Check sheet for the modelled part. Datum: model origin and axes. Units: mm. Give positions to 0.01 mm unless a question says otherwise; leave off trailing zeros. Order: outer loops, then holes, each group sorted by start corner. A loop starts at its lowest first (then second) coordinate and runs counter-clockwise, first axis right, second up. Notation, with made-up numbers: (-37, 37) -> (6, 37) arc R24 cw to (6, 66) -> close; hole circle Ø2 at (63.25, 19.25). An arc over 180 degrees is marked (long way). Write each question's results on one line, items separated by ' | '.
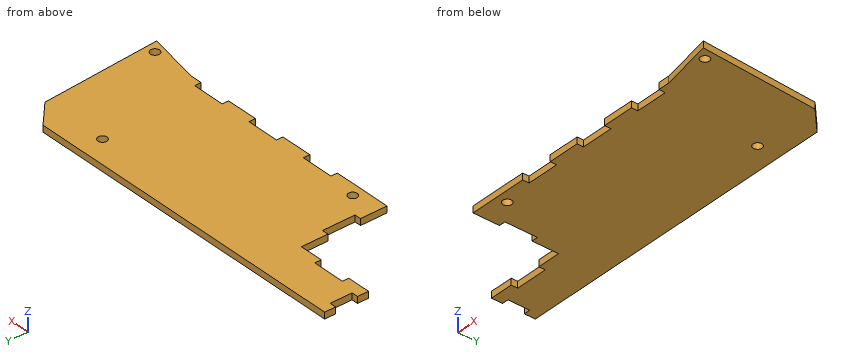
Autodesk Inventor part; units mm, degrees
ref_plane "YZ Plane" through (0, 0, 0) normal (1, 0, 0) x (0, 1, 0)
ref_plane "XZ Plane" through (0, 0, 0) normal (0, 1, 0) x (-1, 0, 0)
ref_plane "XY Plane" through (0, 0, 0) normal (0, 0, 1) x (1, 0, 0)
sketch "Sketch1" plane through (0, 0, 0) normal (0, 0, 1) x (1, 0, 0)
  line L0 (-66.5, -32.75) -> (66.5, -32.75)
  line L1 (66.5, -32.75) -> (66.5, 32.75)
  line L2 (66.5, 32.75) -> (-66.5, 32.75)
  line L3 (-66.5, 32.75) -> (-66.5, -32.75)
  line L4 (-66.5, -32.75) -> (66.5, 32.75) construction
  line L5 (66.5, -32.75) -> (-66.5, 32.75) construction
  line L6 (-103.5, 32.75) -> (-66.5, 32.75)
  line L7 (-66.5, 32.75) -> (-66.5, 12.25)
  line L8 (-66.5, 12.25) -> (-103.5, 12.25)
  line L9 (-103.5, 12.25) -> (-103.5, 32.75)
  line L10 (-103.5, 32.75) -> (-66.5, 12.25) construction
  line L11 (-66.5, 32.75) -> (-103.5, 12.25) construction
  line L12 (66.5, -32.75) -> (61.9198, 32.75)
  circle A0 centre (-53.5, -22.75) radius 2.1
  circle A1 centre (31.5, 22.25) radius 2.1
  line L13 (-66.5, -27.75) -> (41.5, -27.75)
  line L14 (41.5, -27.75) -> (66.5, -32.75)
  circle A2 centre (61.5, -27.75) radius 2.1
  point P0 (0, 0)
  point P1 (-85, 22.5)
  dimension "d0" = 65.5
  dimension "d1" = 133
  dimension "d3" = 37
  dimension "d4" = 4.2
  dimension "d5" = 13
  dimension "d7" = 98
  dimension "d8" = 108
  dimension "d9" = 5
  dimension "d10" = 5
  dimension "d11" = 50
  dimension "d12" = 4.2
  dimension "d13" = 4.2
  dimension "d15" = 5
  dimension "d16" = 4
  dimension "d36" = 40
extrude "Extrusion1" add sketch "Sketch1" along normal blind 3 contours L14 L13 L3 L2 L12 | L8 L9 L6 L3
sketch "Sketch2" plane through (0, 0, 3) normal (0, 0, 1) x (1, 0, 0)
  line L0 (66.5, -32.75) -> (61.9198, 32.75) construction
  line L1 (61.9198, 32.75) -> (-103.5, 32.75) construction
  line L2 (-103.5, 32.75) -> (-103.5, 12.25) construction
  line L3 (-103.5, 12.25) -> (-66.5, 12.25) construction
  line L4 (-66.5, 12.25) -> (-66.5, -27.75) construction
  line L5 (-66.5, -27.75) -> (41.5, -27.75) construction
  line L6 (41.5, -27.75) -> (66.5, -32.75) construction
  circle A0 centre (-53.5, -22.75) radius 2.1 construction
  circle A1 centre (31.5, 22.25) radius 2.1 construction
  circle A2 centre (61.5, -27.75) radius 2.1 construction
  line L7 (-103.5, 27.6) -> (-100.5, 27.6)
  line L8 (-100.5, 27.6) -> (-100.5, 17.4)
  line L9 (-100.5, 17.4) -> (-103.5, 17.4)
  line L10 (-103.5, 17.4) -> (-103.5, 27.6)
  line L11 (-103.5, 27.6) -> (-100.5, 17.4) construction
  line L12 (-100.5, 27.6) -> (-103.5, 17.4) construction
  line L13 (-92.6, 12.25) -> (-77.4, 12.25)
  line L14 (-77.4, 12.25) -> (-77.4, 15.25)
  line L15 (-77.4, 15.25) -> (-92.6, 15.25)
  line L16 (-92.6, 15.25) -> (-92.6, 12.25)
  line L17 (-92.6, 12.25) -> (-77.4, 15.25) construction
  line L18 (-77.4, 12.25) -> (-92.6, 15.25) construction
  line L19 (-103.5, 12.25) -> (-66.5, 12.25)
  line L20 (-66.5, -15.35) -> (-63.5, -15.35)
  line L21 (-63.5, -15.35) -> (-63.5, -0.15)
  line L22 (-63.5, -0.15) -> (-66.5, -0.15)
  line L23 (-66.5, -0.15) -> (-66.5, -15.35)
  line L24 (-66.5, -15.35) -> (-63.5, -0.15) construction
  line L25 (-63.5, -15.35) -> (-66.5, -0.15) construction
  line L26 (-66.5, 12.25) -> (-66.5, -27.75)
  line L27 (-39.1, -27.75) -> (-23.9, -27.75)
  line L28 (-23.9, -27.75) -> (-23.9, -24.75)
  line L29 (-23.9, -24.75) -> (-39.1, -24.75)
  line L30 (-39.1, -24.75) -> (-39.1, -27.75)
  line L31 (-39.1, -27.75) -> (-23.9, -24.75) construction
  line L32 (-23.9, -27.75) -> (-39.1, -24.75) construction
  line L33 (-66.5, -27.75) -> (41.5, -27.75)
  line L34 (-9.1, -27.75) -> (6.1, -27.75)
  line L35 (6.1, -27.75) -> (6.1, -24.75)
  line L36 (6.1, -24.75) -> (-9.1, -24.75)
  line L37 (-9.1, -24.75) -> (-9.1, -27.75)
  line L38 (-9.1, -27.75) -> (6.1, -24.75) construction
  line L39 (6.1, -27.75) -> (-9.1, -24.75) construction
  line L40 (20.9, -27.75) -> (36.1, -27.75)
  line L41 (36.1, -27.75) -> (36.1, -24.75)
  line L42 (36.1, -24.75) -> (20.9, -24.75)
  line L43 (20.9, -24.75) -> (20.9, -27.75)
  line L44 (20.9, -27.75) -> (36.1, -24.75) construction
  line L45 (36.1, -27.75) -> (20.9, -24.75) construction
  point P0 (0, 0)
  point P1 (-102, 22.5)
  point P2 (-103.5, 22.5)
  point P3 (-85, 13.75)
  point P4 (-85, 12.25)
  point P5 (-65, -7.75)
  point P6 (-66.5, -7.75)
  point P7 (-31.5, -26.25)
  point P8 (-1.5, -26.25)
  point P9 (28.5, -26.25)
  point P10 (20.9, -27.75)
  point P11 (36.1, -27.75)
  point P12 (-9.1, -27.75)
  point P13 (6.1, -27.75)
  dimension "d19" = 3
  dimension "d20" = 10.2
  dimension "d21" = 3
  dimension "d22" = 15.2
  dimension "d23" = 3
  dimension "d24" = 15.2
  dimension "d25" = 3
  dimension "d26" = 15.2
  dimension "d27" = 3
  dimension "d28" = 15.2
  dimension "d30" = 35
  dimension "d31" = 3
  dimension "d33" = 15.2
  dimension "d37" = 30
  dimension "d38" = 30
extrude "Extrusion2" cut sketch "Sketch2" against normal through all
chamfer "Chamfer1" distance 10 angle 45 1 edges at (61.9198, 32.75, 1.5)
equation "\"d12\" = d4"
equation "\"d13\" = d12"
equation "\"d21\" = d19"
equation "\"d23\" = d21"
equation "\"d25\" = d23"
equation "\"d27\" = d25"
equation "\"d28\" = d26"
equation "\"d31\" = d27"
equation "\"d33\" = d28"
properties part number "bed_acrylic_side"
1. Section check B-B on y = -22.75. Record the cut outline in (x, z), then the cut area to 3 significant figures.
Verdict:
outline: (-66.5, 0) -> (-55.6, 0) -> (-55.6, 3) -> (-66.5, 3) -> close; (-51.4, 0) -> (65.8, 0) -> (65.8, 3) -> (-51.4, 3) -> close | area: 384 mm^2
2. Section check C-C on z = 0.55. Give the number of separate pieces and of enclosed holes in the cut face, then the cut area to 3 significant figures.
Verdict:
separate pieces: 1 | enclosed holes: 3 | area: 8,370 mm^2
3. Gauge pin test, flat ends, axial feed: pin 1 Ø1.5 at (x, y) = (-76, 23) entering from -Z; pin 2 Ø1.5 at (y, z) = (-19, 1.5) entering from -X; pin 3 Ø1.5 at (y, z) = (-26.5, 1) entering from +X; pin 4 Ø1 at (x, z) = (3, 1) entering from -Y. Record the tip position at first contact, or that the pin passes through.
Verdict:
pin 1: stops at z = 0 | pin 2: stops at x = -66.5 | pin 3: stops at x = 66.12 | pin 4: stops at y = -24.75
4. Material ranges on probe 1 along Y at (x, z) = (-53.5, 1.9); probe 2 along Y at (x, z) = (-64, 1.2); probe 3 along X at (y, z) = (-24.5, 0.5), recorded low to high. Write a range as from..to.
Verdict:
probe 1: y = -27.75..-24.85, -20.65..32.75 | probe 2: y = -27.75..-15.35, -0.15..32.75 | probe 3: x = -66.5..-54.66, -52.34..65.92
5. Section check A-A on x = 31.5. Record the cut outline in (y, z).
Verdict:
outline: (-24.75, 0) -> (20.15, 0) -> (20.15, 3) -> (-24.75, 3) -> close; (24.35, 0) -> (32.75, 0) -> (32.75, 3) -> (24.35, 3) -> close
6. Section check D-D on x = 49. Record the cut outline in (y, z), then the cut area to 3 significant figures.
Verdict:
outline: (-29.25, 0) -> (32.75, 0) -> (32.75, 3) -> (-29.25, 3) -> close | area: 186 mm^2
